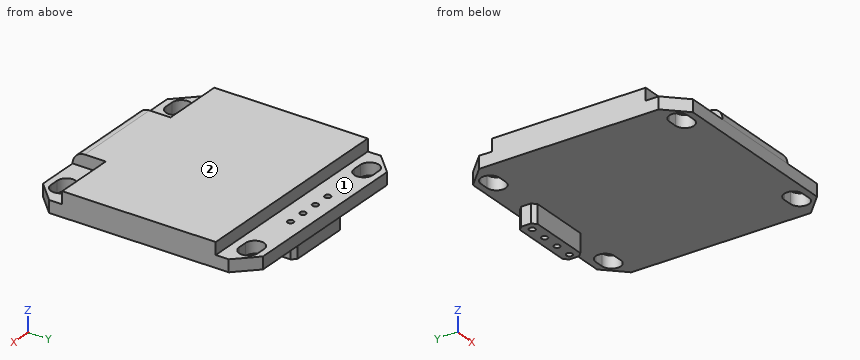
from build123d import *

# Parameters (mm, degrees)
ESQUISSE1_R        = 0.375
BOSS_EXTRU_1_DEPTH = 1.5
BOSS_EXTRU_2_DEPTH = 1.5
CONG_1_R           = 1.5
ESQUISSE3_R        = 0.375
BOSS_EXTRU_3_DEPTH = 2.3


with BuildPart() as part:
    # Esquisse1 → Boss.-Extru.1 (new body)
    with BuildSketch(Plane.XY):
        Polygon((0, -1.46), (2.5, -3.96), (24.5, -3.96), (27, -1.46), (27, 20.76), (24.5, 23.26), (2.5, 23.26), (0, 20.76), align=None)
        with Locations((10.2, 21.3)):
            Circle(ESQUISSE1_R, mode=Mode.SUBTRACT)
        with Locations((12.4, 21.3)):
            Circle(ESQUISSE1_R, mode=Mode.SUBTRACT)
        with Locations((14.6, 21.3)):
            Circle(ESQUISSE1_R, mode=Mode.SUBTRACT)
        with Locations((16.8, 21.3)):
            Circle(ESQUISSE1_R, mode=Mode.SUBTRACT)
        with BuildLine():
            Line((2.75, 22.45), (3.85, 22.45))
            ThreePointArc((3.85, 22.45), (5, 21.3), (3.85, 20.15))
            Line((3.85, 20.15), (2.75, 20.15))
            ThreePointArc((2.75, 20.15), (1.6, 21.3), (2.75, 22.45))
        make_face(mode=Mode.SUBTRACT)
        with BuildLine():
            Line((24.25, 22.45), (23.15, 22.45))
            ThreePointArc((23.15, 22.45), (22, 21.3), (23.15, 20.15))
            Line((23.15, 20.15), (24.25, 20.15))
            ThreePointArc((24.25, 20.15), (25.4, 21.3), (24.25, 22.45))
        make_face(mode=Mode.SUBTRACT)
        with BuildLine():
            Line((24.25, -3.15), (23.15, -3.15))
            ThreePointArc((23.15, -3.15), (22, -2), (23.15, -0.85))
            Line((23.15, -0.85), (24.25, -0.85))
            ThreePointArc((24.25, -0.85), (25.4, -2), (24.25, -3.15))
        make_face(mode=Mode.SUBTRACT)
        with BuildLine():
            Line((2.75, -3.15), (3.85, -3.15))
            ThreePointArc((3.85, -3.15), (5, -2), (3.85, -0.85))
            Line((3.85, -0.85), (2.75, -0.85))
            ThreePointArc((2.75, -0.85), (1.6, -2), (2.75, -3.15))
        make_face(mode=Mode.SUBTRACT)
    extrude(amount=BOSS_EXTRU_1_DEPTH)

    # Esquisse2 → Boss.-Extru.2 (add)
    with BuildSketch(Plane.XY.offset(1.5)):
        Polygon((0, 19.15), (27, 19.15), (27, 0.15), (19.25, 0.15), (19.25, -3.96), (7.75, -3.96), (7.75, 0.15), (0, 0.15), align=None)
    extrude(amount=BOSS_EXTRU_2_DEPTH)

    # Congé1
    cong_1_edges = [part.edges().sort_by_distance(p)[0] for p in [
        (13.5, -3.96, 3),
    ]]
    fillet(cong_1_edges, radius=CONG_1_R)

    # Esquisse3 → Boss.-Extru.3 (add)
    with BuildSketch(Plane(origin=(0, 0, 0), x_dir=(-1, 0, 0), z_dir=(0, 0, -1))):
        Polygon((-17.65, 20.7), (-17.15, 20.2), (-15.45, 20.2), (-13.5, 20.2), (-11.3, 20.2), (-9.6, 20.2), (-9.1, 20.7), (-9.1, 21.9), (-9.6, 22.4), (-11.3, 22.4), (-13.5, 22.4), (-15.45, 22.4), (-17.15, 22.4), (-17.65, 21.9), align=None)
        with Locations((-10.2, 21.3)):
            Circle(ESQUISSE3_R, mode=Mode.SUBTRACT)
        with Locations((-16.8, 21.3)):
            Circle(ESQUISSE3_R, mode=Mode.SUBTRACT)
        with Locations((-12.4, 21.3)):
            Circle(ESQUISSE3_R, mode=Mode.SUBTRACT)
        with Locations((-14.6, 21.3)):
            Circle(ESQUISSE3_R, mode=Mode.SUBTRACT)
    extrude(amount=BOSS_EXTRU_3_DEPTH)


solid = part.part
Work out the finished part from the listing and answer in its coordinate system (mm). Face numbers are marked on the shaded views. A direction names the side the tool comes from. Give positions to 0.01 mm unless a question says otherwise; leave off trailing zeros. Order: outer loops, then holes, each group sorted by start corner. A loop starts at its lowest first (then second) coordinate and runs counter-clockwise, first axis right, second up. Notation, with made-up numbers: (29.25, -27.5) -> (71.25, -27.5) arc R11 ccw to (71.25, -9.5) -> close; hole circle Ø5 at (8.25, 10.5). An arc over 180 degrees is marked (long way). One line per item, written item: value.
Item 1: Straight lines are drawn through the part: probe 1 along X at (y, z) = (21.3, -0.9) (3 decimals); probe 2 along Y at (x, z) = (10.2, -1.3) (3 decimals); probe 3 along Y at (x, z) = (12.4, 0.3) (3 decimals). For each, find the intervals that lie inside material, in ascending order.
Answer sheet:
probe 1: 9.1 to 9.825, 10.575 to 12.025, 12.775 to 14.225, 14.975 to 16.425, 17.175 to 17.65
probe 2: 20.2 to 20.925, 21.675 to 22.4
probe 3: -3.96 to 20.925, 21.675 to 23.26
Item 2: Find section C-C, the plane z = -0.4. Give the vertices of the cut face in (x, y) (3 decimals).
Answer sheet:
outline: (9.1, 20.7) -> (9.6, 20.2) -> (17.15, 20.2) -> (17.65, 20.7) -> (17.65, 21.9) -> (17.15, 22.4) -> (9.6, 22.4) -> (9.1, 21.9) -> close; hole circle Ø0.75 at (10.2, 21.3); hole circle Ø0.75 at (12.4, 21.3); hole circle Ø0.75 at (14.6, 21.3); hole circle Ø0.75 at (16.8, 21.3)
Item 3: Find section A-A, the plane y = 21.3. State how many separate pieces and enclosed holes the cut face has, plus the area to 3 significant figures.
Answer sheet:
separate pieces: 7
enclosed holes: 0
area: 36.9 mm²
Item 4: Flat-ended cylindrical pins translate along their axes: P1, Ø1.5, axis at x = 4.5, z = 2.5, coming from the +Y side; P2, Ø3.5, axis at x = 19, y = 21, coming from the +Z side; P3, Ø0.8, axis at x = 23, z = 2.5, coming from the -Y side. Find the tip coordinate at first contact, or state that the pin passes through.
Answer sheet:
P1: y = 19.15
P2: z = 1.5
P3: y = 0.15
Item 5: Find section B-B, the plane x = 3.25. Give the vertices of the cut face in (y, z), plus the area to 3 significant figures.
Answer sheet:
outline: (-3.96, 0) -> (-3.15, 0) -> (-3.15, 1.5) -> (-3.96, 1.5) -> close; (-0.85, 0) -> (20.15, 0) -> (20.15, 1.5) -> (19.15, 1.5) -> (19.15, 3) -> (0.15, 3) -> (0.15, 1.5) -> (-0.85, 1.5) -> close; (22.45, 0) -> (23.26, 0) -> (23.26, 1.5) -> (22.45, 1.5) -> close
area: 62.4 mm²
Item 6: Find section D-D, the plane y = -2. Give the vertices of the cut face in (x, z).
Answer sheet:
outline: (0.54, 0) -> (1.6, 0) -> (1.6, 1.5) -> (0.54, 1.5) -> close; (5, 0) -> (22, 0) -> (22, 1.5) -> (19.25, 1.5) -> (19.25, 3) -> (7.75, 3) -> (7.75, 1.5) -> (5, 1.5) -> close; (25.4, 0) -> (26.46, 0) -> (26.46, 1.5) -> (25.4, 1.5) -> close
Item 7: A tool of negligible diameter and unlimited length cuts with its end or side. For the marked faces 1 and 2, from which of +Z, -Z, +X, -X, +Y, -Y can it reach the whole face along a straight path? Write none if from no direction.
Answer sheet:
face 1: +Z, +X, -X, +Y
face 2: +Z, +X, -X, +Y, -Y
